For this review, take the finished solid that the model builds, in its own axes (mm). A direction names the side the tool comes from. Round coordinates to 2 decimals unless told otherwise and drop trailing zeros. Order: outer loops, then holes, each group sorted by start corner. A loop starts at its lowest first (then second) coordinate and runs counter-clockwise, first axis right, second up.
from build123d import *

# Parameters (mm, degrees)
PAD019_DEPTH    = 5
SKETCH047_W     = 7.74745
SKETCH047_H     = 7
POCKET015_DEPTH = 7
SKETCH048_R     = 1.6
POCKET016_DEPTH = 5


with BuildPart() as part:
    # Sketch046 → Pad019 (new body, symmetric)
    with BuildSketch(Plane.YZ):
        Polygon((13.031275, 70.374863), (10.236371, 70.374863), (1.084429, 61.39085), (13.031275, 61.39085), align=None)
    extrude(amount=PAD019_DEPTH, both=True)

    # Sketch047 (on DatumPlane) → Pocket015 (cut)
    with BuildSketch(Plane(origin=(0, 0, 71.374863), x_dir=(0, -1, 0), z_dir=(0, 0, 1))):
        with Locations((-6.354073, 0)):
            Rectangle(SKETCH047_W, SKETCH047_H)
    extrude(amount=-POCKET015_DEPTH, mode=Mode.SUBTRACT)

    # Sketch048 (on Face9 of Pocket015) → Pocket016 (cut)
    with BuildSketch(Plane(origin=(0, 10.227798, 0), x_dir=(0, 0, -1), z_dir=(0, -1, 0))):
        with Locations((-67.397021, 0)):
            Circle(SKETCH048_R)
    extrude(amount=-POCKET016_DEPTH, mode=Mode.SUBTRACT)


with BuildPart() as part_1:
    # Body021 placement: moved
    add(part.part.moved(Location((20, 0, 0))))


with BuildPart() as part_2:
    # Body022 placement: moved
    add(part_1.part.moved(Location((-40, 0, 0))))


solid = part_2.part
(1) Clearance check with flat-ended pins moving along their axes: P1, Ø3, axis at x = -19.5, z = 68, coming from the -Y side; P2, Ø2, axis at y = 2.5, z = 64.5, coming from the +X side. State where each tip first meets the part, or that it passes through.
(2) Add section C-C on y = 6.75. Give the boundary of the cut face in (x, z), plus the area to 3 significant figures.
(3) Draft analysis for pull direction Z (two halves, no side actions). For faces 3 (the face through (-25, 8, 65)), 4 (the face through (-18.414, 11.61, 67.605)), 5 (the face through (-20, 7, 61.391)), state which applies: pulls with the +Z half, pulls with the -Z half, needs draft (parallel to the pull), parting line crosses it, or undercut.
(4) Wall thickness on L1, parallel to Y at x = -19.25, z = 70; L2, parallel to Z at x = -20.5, y = 11.25; L3, parallel to Z at x = -19.75, y = 9.75: over which ranges is each line inside the solid? List them lowest first.
(5) Tool access review of faces 1 (the face through (-22, 10.228, 67)), 2 (the face through (-19.93, 3.69, 63.95)): name each direction out of +Z, -Z, +X, -X, +Y, -Y from which nothing blocks a thin tool from reaching the whole face with its end or side.
(6) Add section B-B on z = 65.25. Give the boundary of the cut face in (x, y).
Here are the results:
1. P1: stops at y = 10.23
1. P2: passes through
2. outline: (-25, 61.39) - (-15, 61.39) - (-15, 66.95) - (-16.5, 66.95) - (-16.5, 64.37) - (-23.5, 64.37) - (-23.5, 66.95) - (-25, 66.95) - close
2. area: 37.6 mm2
3. face 3: needs draft
3. face 4: undercut
3. face 5: pulls with the -Z half
4. L1: y = 10.23 to 13.03
4. L2: z = 61.39 to 65.88, 68.92 to 70.37
4. L3: z = 61.39 to 64.37
5. face 1: +Z, -Y
5. face 2: +Z, +X, -X, -Y
6. outline: (-25, 5.02) - (-23.5, 5.02) - (-23.5, 10.23) - (-16.5, 10.23) - (-16.5, 5.02) - (-15, 5.02) - (-15, 13.03) - (-25, 13.03) - close
